Here's how the part is built. I have some questions about the finished solid (model axes, mm). A direction names the side the tool comes from. Coordinates: 2 decimals unless noted, no trailing zeros. Loops run counter-clockwise (first coordinate to the right, second up) from the corner with the lowest first, then second, coordinate; pieces in that order, holes last. Notation, with made-up numbers: (89, 69) -> (119, 69) arc R19 cw to (119, 103) -> close; hole circle Ø3 at (89, -27). An arc over 180 degrees is marked (long way). Answer as a JSON object with one key per item and string values. Group by question number.
1) I'm going to push flat-ended pins straight in: pin 1 (2 mm diameter, centred on x = -50.5, z = -2.5, fed in from -Y); pin 2 (1.5 mm diameter, centred on y = 8.5, z = -5, fed in from +X); pin 3 (1.2 mm diameter, centred on y = -29.5, z = -2, fed in from +X). Where does each tip first touch, or does it pass through?
2) I need wall thicknesses on probe 1 along Y at (x, z) = (-58, -3); probe 2 along X at (y, z) = (-20, -0.75); probe 3 along X at (y, z) = (-24.5, -2). Which ranges of each line are inside material? Lowest first, please. Write a range as [from, to].
3) Which directions (+Z, -Z, +X, -X, +Y, -Y) give clear straight access to the entire face, cutting with the end or side of a thin tool? Please do faces 4 (the flat face through (-52.1, -5, -5.4)), 5 (the flat face through (-2, 13, -3)), 6 (the flat face through (11, -0.5, -7.2)), 7 (the flat face through (-15, 25, -3)).
4) I want a section at B-B (x = -11). Write out the boundary of the cut face in (y, z), then the cut area to 3 significant figures.
5) I want a section at C-C (z = -2.5). Count the separate pieces of the cut face and the enclosed holes in it, then the cut area to 3 significant figures.
6) I want a section at D-D (y = 10). Write out the boundary of the cut face in (x, z).
7) If we mould it in two halves opening along Y, with no side actions, what happens to faces 1 (the flat face through (-27, -37, -5)), 2 (the flat face through (-34, 1, 0)), 3 (the flat face through (-6, 30, -2))? For each: +Y half, -Y half, draft (parallel to the pull), parting line (faces both ways), or undercut.
8) I want a section at A-A (y = -30). Write out the boundary of the cut face in (x, z), then the cut area to 3 significant figures.
```python
from build123d import *

# Parameters (mm, degrees)
F0_R     = 4
F0_W     = 11
F0_H     = 74
F0_W_2   = 17
F0_H_2   = 4
F1_DEPTH = 10
F5_DEPTH = 7


with BuildPart() as f1:
    # F0 (on Top) → F1 (new body)
    with BuildSketch(Plane.XY):
        Polygon((-47, -37), (-20, -37), (-20, 13), (-20, 37), (-47, 37), (-47, 29), (-44.5, 29), (-44.5, 5), (-47, 5), (-47, 0), (-47, -5), (-44.5, -5), (-44.5, -29), (-47, -29), align=None)
        Polygon((-9, -37), (-9, -13), (11, -13), (11, 13), (-15, 13), (-15, 37), (-20, 37), (-20, 13), (-20, -37), align=None)
        Circle(F0_R, mode=Mode.SUBTRACT)
        with Locations((-57.5, 0)):
            Rectangle(F0_W, F0_H)
        Polygon((-15, 13), (11, 13), (11, 30), (-6, 30), (-6, 34), (11, 34), (11, 37), (-15, 37), align=None)
        Polygon((-52, -37), (-47, -37), (-47, -29), (-44.5, -29), (-44.5, -5), (-47, -5), (-47, 0), (-47, 5), (-44.5, 5), (-44.5, 29), (-47, 29), (-47, 37), (-52, 37), align=None)
        Polygon((11, -13), (-9, -13), (-9, -37), (11, -37), (11, -34), (-6, -34), (-6, -30), (11, -30), align=None)
        with Locations((2.5, 32)):
            Rectangle(F0_W_2, F0_H_2)
        with Locations((2.5, -32)):
            Rectangle(F0_W_2, F0_H_2)
        Circle(F0_R)
    extrude(amount=-F1_DEPTH)

    # F0 (on Top) → F2 (revolve, cut)
    with BuildSketch(Plane.XY):
        Polygon((-52, -37), (-47, -37), (-47, -29), (-44.5, -29), (-44.5, -5), (-47, -5), (-47, 0), (-47, 5), (-44.5, 5), (-44.5, 29), (-47, 29), (-47, 37), (-52, 37), align=None)
    revolve(axis=Axis((-52, 0, 0), (0, -1, 0)), mode=Mode.SUBTRACT)

    # F0 (on Top) → F3 (revolve, cut)
    with BuildSketch(Plane.XY):
        with Locations((2.5, 32)):
            Rectangle(F0_W_2, F0_H_2)
    revolve(axis=Axis((2.5, 30, 0), (1, 0, 0)), mode=Mode.SUBTRACT)

    # F0 (on Top) → F4 (revolve, cut)
    with BuildSketch(Plane.XY):
        with Locations((2.5, -32)):
            Rectangle(F0_W_2, F0_H_2)
    revolve(axis=Axis((2.5, -30, 0), (1, 0, 0)), mode=Mode.SUBTRACT)

    # F0 (on Top) → F5 (cut)
    with BuildSketch(Plane.XY):
        Polygon((-9, -37), (-9, -13), (11, -13), (11, 13), (-15, 13), (-15, 37), (-20, 37), (-20, 13), (-20, -37), align=None)
        Circle(F0_R, mode=Mode.SUBTRACT)
    extrude(amount=-F5_DEPTH, mode=Mode.SUBTRACT)


solid = f1.part
```
Determined:
{
 "1": {"pin 1": "through", "pin 2": "x = -20", "pin 3": "x = -6"},
 "2": {"probe 1": "[-37, -29], [-5, 5], [29, 37]", "probe 2": "[-63, -59.46], [-44.54, -20], [-9, 11]", "probe 3": "[-63, -59.23], [-44.77, -20], [-9, 11]"},
 "3": {"face 4": "+Z", "face 5": "+Z, +X", "face 6": "+Z, -Z, +X, +Y, -Y", "face 7": "+Z, +Y, -Y"},
 "4": {"outline": "(-37, -10) -> (37, -10) -> (37, 0) -> (13, 0) -> (13, -7) -> (-37, -7) -> close", "area": "390 mm^2"},
 "5": {"separate pieces": "5", "enclosed holes": "0", "area": "3,220 mm^2"},
 "6": {"outline": "(-63, -10) -> (11, -10) -> (11, -7) -> (-20, -7) -> (-20, 0) -> (-44.5, 0) arc R7.5 cw to (-59.5, 0) -> (-63, 0) -> close"},
 "7": {"face 1": "-Y half", "face 2": "draft", "face 3": "undercut"},
 "8": {"outline": "(-63, -10) -> (11, -10) -> (11, -4) -> (-6, -4) -> (-6, 0) -> (-9, 0) -> (-9, -7) -> (-20, -7) -> (-20, 0) -> (-47, 0) arc R5 cw to (-57, 0) -> (-63, 0) -> close", "area": "556 mm^2"}
}
